Input: part model. Units: mm. Frame: model coordinates. Face numbers are marked on the shaded views. A direction names the side the tool comes from. Coordinates: 2 decimals unless noted, no trailing zeros. Write each loop counter-clockwise with the first axis right and the second up, starting at its lowest first coordinate (ties: lowest second). Pieces come first, ordered by that corner, then holes. Notation, with made-up numbers: (51, 50) - (103, 50) arc R11 ccw to (103, 58) - close; hole circle Ø9 at (5.25, 84). An arc over 180 degrees is marked (long way). Use CSV: the item, a comma, the result in double quotes.
```python
from build123d import *


with BuildPart() as part:
    # Sketch1 → Revolve1 (revolve)
    with BuildSketch(Plane.XY):
        with BuildLine():
            Line((-49.784, 0), (-39.839899999, 0))
            ThreePointArc((-39.839899999, 0), (-38.717367984, -0.464967985), (-38.252399999, -1.5875))
            Line((-38.252399999, -1.5875), (-38.2524, -17.4625))
            Line((-38.2524, -17.4625), (-35.0774, -17.4625))
            Line((-35.0774, -17.4625), (-35.0774, -3.175))
            ThreePointArc((-35.0774, -3.175), (-34.14746403, -0.92993597), (-31.9024, 0))
            Line((-31.9024, 0), (-5.588, 0))
            Line((-5.588, 0), (-5.588, 9.906))
            Line((-5.588, 9.906), (-8.763, 9.906))
            ThreePointArc((-8.763, 9.906), (-11.70403388, 8.68778388), (-12.92225, 5.74675))
            ThreePointArc((-12.92225, 5.74675), (-14.14046612, 2.80571612), (-17.0815, 1.5875))
            Line((-17.0815, 1.5875), (-49.784, 1.5875))
            Line((-49.784, 1.5875), (-49.784, 0))
        make_face()
    revolve(axis=Axis((0, 55, 0), (0, -1, 0)))

    # Sketch5 → 1/4 NPT Tapped Hole1 (revolve, cut)
    with BuildSketch(Plane(origin=(0, 9.906, 0), x_dir=(0, 0, 1), z_dir=(1, 0, 0))):
        Polygon((0, 0), (0, 27.3685), (5.5626, 27.3685), (5.5626, 9.906), (6.557984794, 9.906), (6.8545837, 0), align=None)
    revolve(axis=Axis((0, 16.256, 0), (0, -1, 0)), mode=Mode.SUBTRACT)


solid = part.part
```
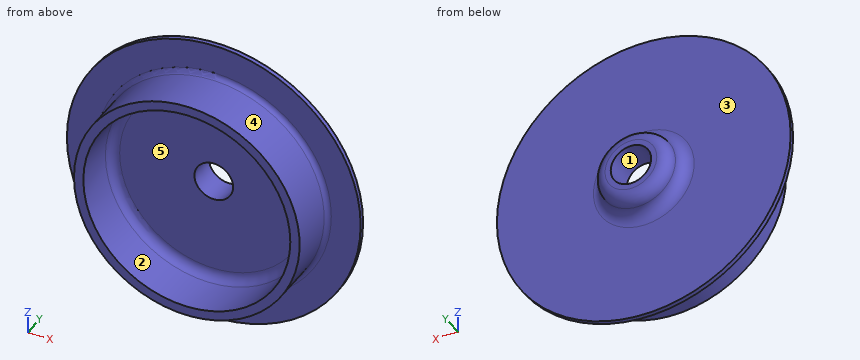
(1) Draft query along X for the marked faces 3, 4 and 5. Return one class per face: pulls with the +X half, pulls with the -X half, needs draft (parallel to the pull), parting line crosses it, or undercut.
Check values:
face 3,"needs draft"
face 4,"parting line crosses it"
face 5,"undercut"
(2) Reachability of the marked faces 1 and 2 from +Z, -Z, +X, -X, +Y, -Y: full face, straight path, thin tool, end or side. Return the list, or none.
Check values:
face 1,"+Y"
face 2,"-Y"
(3) Cut plane B-B on y = 4.5. Return loops of the section in (x, z).
Check values:
outline,"circle Ø26.23 at (0, 0); hole circle Ø13.39 at (0, 0)"
(4) Pin query (flat end, axial travel): pin 1 Ø12 at (y, z) = (-2, 32) entering from +X; pin 2 Ø12 at (x, y) = (5, -0.5) entering from -Z; pin 3 Ø1 at (y, z) = (-7.5, 10) entering from +X. Return the tip coordinate at first contact, or that it passes through.
Check values:
pin 1,"x = 42.24"
pin 2,"z = -49.78"
pin 3,"x = 37.05"
(5) Cut plane A-A on y = -9.5. Return loops of the section in (x, z).
Check values:
outline,"circle Ø76.5 at (0, 0); hole circle Ø70.15 at (0, 0)"
(6) Ray query, probe 1 along X at (y, z) = (-11.5, 0); probe 2 along Y at (x, z) = (-15, 14). Return the intervals inside material, ascending. Write a range as from..to.
Check values:
probe 1,"-38.25..-35.08, 35.08..38.25"
probe 2,"0..1.59"
